The drawing under review shows one solid part. Ordinate dimensions are in mm from its lowest x, y, z. Give positions to 0.01 mm unless a question says otherwise; leave off trailing zeros. Answer as a JSON object with one key per item and string values.
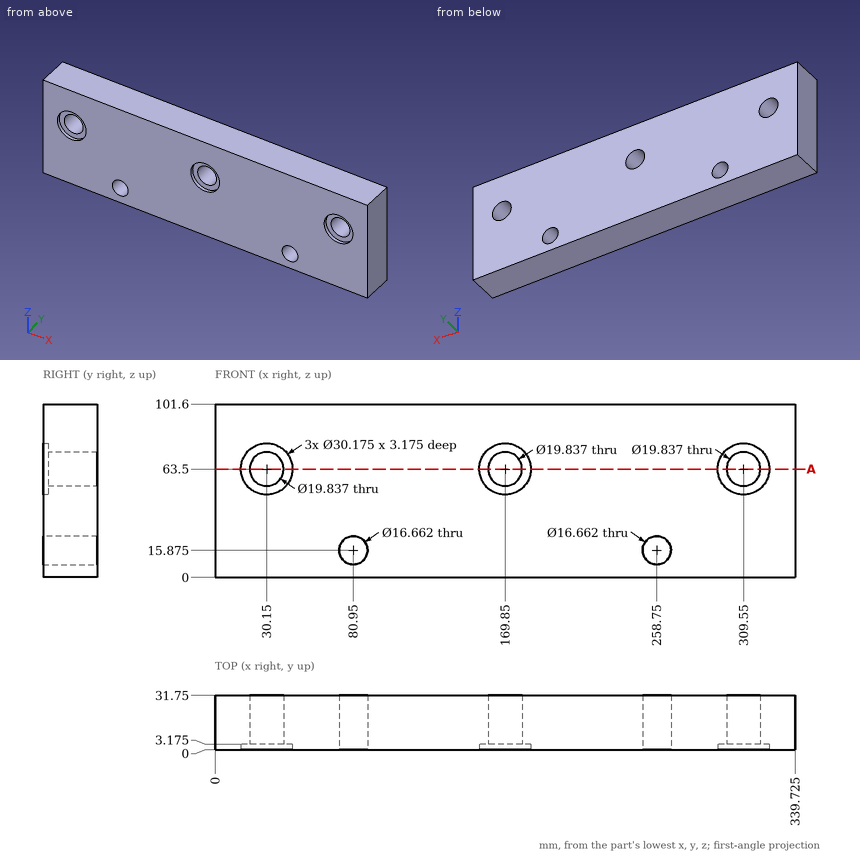
(1) We need section A-A, the plane z = 63.5. Give the number of separate pieces and of enclosed holes in the cut face, then the cut area to 3 significant figures.
Here are the results:
{"separate pieces": "4", "enclosed holes": "0", "area": "8,800 mm²"}
(2) Clearance check with flat-ended pins moving along their axes: pin 1 (4 mm diameter, centred on x = 57.5, y = 8.5, fed in from -Z); pin 2 (16 mm diameter, centred on x = 169.85, z = 63.5, fed in from -Y); pin 3 (15 mm diameter, centred on x = 36, z = 67, fed in from -Y) (3 decimals). State where each tip first meets the part, or that it passes through.
Here are the results:
{"pin 1": "stops at z = 0", "pin 2": "passes through", "pin 3": "stops at y = 3.175"}
(3) For line 1 along X through (y, z) = (1, 63) (1 decimal); line 2 along X through (y, z) = (25.75, 63.5) (1 decimal); line 3 along X through (y, z) = (9, 18) (1 decimal), list the stretches that pass through material, from the lowest coordinate up.
Here are the results:
{"line 1": "x = 0 to 15.1, 45.2 to 154.8, 184.9 to 294.5, 324.6 to 339.7", "line 2": "x = 0 to 20.2, 40.1 to 159.9, 179.8 to 299.6, 319.5 to 339.7", "line 3": "x = 0 to 72.9, 89 to 250.7, 266.8 to 339.7"}
